```python
from build123d import *

# Parameters (mm, degrees)
SKETCH1_R           = 16.5
BOSS_EXTRUDE1_DEPTH = 7.25
SKETCH2_R           = 2.05
CUT_EXTRUDE1_DEPTH  = 48.105394919
SKETCH9_R           = 11.5
CUT_EXTRUDE2_DEPTH  = 6.25


with BuildPart() as part:
    # Sketch1 → Boss-Extrude1 (new body)
    with BuildSketch(Plane(origin=(0, 0, 0), x_dir=(1, 0, 0), z_dir=(0, 1, 0))):
        with Locations(Location((-11.073338277, 20.997556543, 0), (0, 0, 90))):
            Circle(SKETCH1_R)
    extrude(amount=BOSS_EXTRUDE1_DEPTH)

    # Sketch2 → Cut-Extrude1 (cut, through all)
    with BuildSketch(Plane(origin=(0, 7.25, 0), x_dir=(1, 0, 0), z_dir=(0, 1, 0))):
        with Locations(Location((-11.112077012, 20.900709706, 0), (0, 0, 270))):
            Circle(SKETCH2_R)
    extrude(amount=-CUT_EXTRUDE1_DEPTH, mode=Mode.SUBTRACT)

    # Sketch9 → Cut-Extrude2 (cut)
    with BuildSketch(Plane(origin=(0, 7.25, 0), x_dir=(1, 0, 0), z_dir=(0, 1, 0))):
        with Locations(Location((-11.112077012, 20.900709706, 0), (0, 0, 270))):
            Circle(SKETCH9_R)
    extrude(amount=-CUT_EXTRUDE2_DEPTH, mode=Mode.SUBTRACT)


solid = part.part
```
Work out the finished part from the listing and answer in its coordinate system (mm). A direction names the side the tool comes from. Give positions to 0.01 mm unless a question says otherwise; leave off trailing zeros. Loops run counter-clockwise (first coordinate to the right, second up) from the corner with the lowest first, then second, coordinate; pieces in that order, holes last. Notation, with made-up numbers: (-36.5, 86.25) -> (-4.5, 86.25) arc R24 ccw to (-4.5, 117.25) -> close; hole circle Ø2 at (-21, 63.5). An arc over 180 degrees is marked (long way). Use CSV: the item, a comma, the result in double quotes.
1. The mould has two halves that part along X. Classify faces 3 (the cylindrical face through (-4.754, 3.574, -36.239)), 4 (the flat face through (-15, 7.25, -32)), 5 (the cylindrical face through (-11.02, 0.51, -22.95)): +X half, -X half, draft (parallel to the pull), parting line (faces both ways), or undercut.
Found:
face 3,"parting line"
face 4,"draft"
face 5,"undercut"
2. The part is cut by section D-D (y = 2.25). Write down the section's boundary in (x, z), then the cut area to 3 significant figures.
Found:
outline,"circle Ø33 at (-11.07, -21); hole circle Ø23 at (-11.11, -20.9)"
area,"440 mm^2"
3. A tool of negligible diameter and unlimited length cuts with its end or side. For faces 1 (the flat face through (-11, 0, -24)), 2 (the cylindrical face through (-15.52, 4.17, -10.28)), from which of +Z, -Z, +X, -X, +Y, -Y can it reach the whole face along a straight path? Write none if from no direction.
Found:
face 1,"+Z, -Z, +X, -X, -Y"
face 2,"+Y"
4. Flat-ended cylindrical pins translate along their axes: pin 1 Ø1 at (y, z) = (2.5, -24) entering from -X; pin 2 Ø4 at (x, y) = (-8, 1) entering from +Z. Find the tip coordinate at first contact, or state that the pin passes through.
Found:
pin 1,"x = -27.38"
pin 2,"z = -4.53"
5. The part is cut by section A-A (z = -19.5). Write down the section's boundary in (x, y), then the cut area to 3 significant figures.
Found:
outline,"(-27.51, 0) -> (-12.61, 0) -> (-12.61, 1) -> (-22.53, 1) -> (-22.53, 7.25) -> (-27.51, 7.25) -> close; (-9.62, 0) -> (5.36, 0) -> (5.36, 7.25) -> (0.3, 7.25) -> (0.3, 1) -> (-9.62, 1) -> close"
area,"92.6 mm^2"
6. The part is cut by section B-B (x = -20). Write down the section's boundary in (y, z).
Found:
outline,"(0, -34.87) -> (7.25, -34.87) -> (7.25, -28.2) -> (1, -28.2) -> (1, -13.6) -> (7.25, -13.6) -> (7.25, -7.12) -> (0, -7.12) -> close"
7. Straight lines are drawn through the part: line 1 (X direction, y = 1.75, z = -21); line 2 (Z direction, x = -11, y = 6.25); line 3 (Y direction, x = -5, z = -28.5). For each, find the intervals that lie inside material, in ascending order.
Found:
line 1,"-27.57 to -22.61, 0.39 to 5.43"
line 2,"-37.5 to -32.4, -9.4 to -4.5"
line 3,"0 to 1"
8. The part is cut by section C-C (z = -14.5). Write down the section's boundary in (x, y).
Found:
outline,"(-26.24, 0) -> (4.09, 0) -> (4.09, 7.25) -> (-1.56, 7.25) -> (-1.56, 1) -> (-20.67, 1) -> (-20.67, 7.25) -> (-26.24, 7.25) -> close"
